Autodesk Inventor part; units mm, degrees
ref_plane "YZ Plane" through (0, 0, 0) normal (1, 0, 0) x (0, 1, 0)
ref_plane "XZ Plane" through (0, 0, 0) normal (0, 1, 0) x (-1, 0, 0)
ref_plane "XY Plane" through (0, 0, 0) normal (0, 0, 1) x (1, 0, 0)
sketch "Sketch1" plane through (0, 0, 0) normal (0, 0, 1) x (1, 0, 0)
  line L0 (0, 0) -> (43.269, 0)
  line L1 (43.269, 0) -> (43.269, 50)
  line L2 (43.269, 50) -> (50, 50)
  line L3 (50, 50) -> (50, 20)
  line L4 (50, 20) -> (43.269, 20)
  line L5 (43.269, 20) -> (43.269, 50)
  line L6 (3.269, 3.269) -> (23.269, 3.269)
  line L7 (23.269, 3.269) -> (23.269, 10)
  line L8 (23.269, 10) -> (3.269, 10)
  line L9 (3.269, 10) -> (3.269, 3.269)
  line L10 (0, 10) -> (3.269, 10)
  line L11 (23.269, 10) -> (43.269, 10)
  line L12 (43.269, 50) -> (40, 50)
  line L13 (0, 10) -> (0, 0)
  line L14 (0, 10) -> (0, 13.269)
  line L15 (0, 13.269) -> (40, 50)
  point P0 (13.269, 3.269)
  point P1 (13.269, 0)
  dimension "d2" = 30
  dimension "d3" = 20
  dimension "d5" = 6.731
  dimension "d6" = 10
  dimension "d9" = 3.269
  dimension "d11" = 20
  dimension "d12" = 20
  dimension "d14" = 3.269
  dimension "d15" = 3.269
extrude "Extrusion1" add sketch "Sketch1" along normal blind 6.731 contours L13 L10 L9 L6 L7 L11 L1 L0 | L14 L15 L12 L1 L11 L8 L10 | L1 L2 L3 L4
fillet "Fillet1" radius 2 3 edges at (40, 50, 3.3655) (0, 13.269, 3.3655) (0, 0, 3.3655)
equation "\"d5\" = THICKB"
equation "\"d7\" = THICKB"
equation "\"THICKA\" = 3.175"
equation "\"THICKB\" = 6.731"
equation "\"THICKC\" = 12.7"
equation "\"THICKPLY\" = 5"
equation "\"MAGDIA\" = 9.5"
equation "\"BALLDIA\" = 12"
properties part number "Mount_Mega_End"
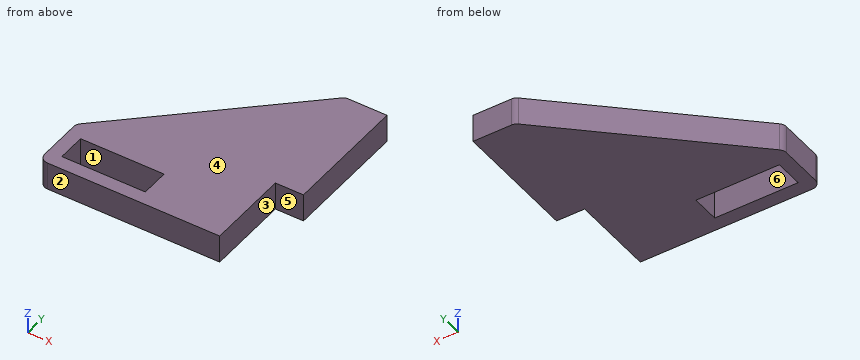
Can you work these out from the model? Positions are in its coordinate system, mm. Face numbers are marked on the shaded views. A direction names the side the tool comes from. Give positions to 0.01 mm unless a question says otherwise; leave off trailing zeros. Loops run counter-clockwise (first coordinate to the right, second up) from the corner with the lowest first, then second, coordinate; pieces in that order, holes last. Notation, with made-up numbers: (60, 39) - (116, 39) arc R4 cw to (116, 45) - close; hole circle Ø2 at (-35.5, 44). An arc over 180 degrees is marked (long way). Answer as a JSON object with one key per item and string values.
Q1. Will these pins go through, and if not, where does the flat tip stop? P1, Ø3.5, axis at y = 8, z = 2.5, coming from the +X side; P2, Ø3.5, axis at x = 17.5, z = 2.5, coming from the +Y side; P3, Ø12, axis at x = 6, y = 31.5, coming from the +Z side; P4, Ø4, axis at y = 20, z = 3, coming from the -X side.
Geometry says:
{"P1": "x = 43.27", "P2": "y = 30.95", "P3": "through", "P4": "x = 5.15"}
Q2. Imagine slicing it at A-A on z = 4.5. Write out the boundary of the cut face in (x, y).
Geometry says:
{"outline": "(0, 2) arc R2 ccw to (2, 0) - (43.27, 0) - (43.27, 20) - (50, 20) - (50, 50) - (40.78, 50) arc R2 ccw to (39.43, 49.47) - (0.65, 13.86) arc R2 ccw to (0, 12.39) - close; hole (3.27, 3.27) - (23.27, 3.27) - (23.27, 10) - (3.27, 10) - close"}
Q3. Imagine slicing it at D-D on x = 24.5. Write out the boundary of the cut face in (y, z).
Geometry says:
{"outline": "(0, 0) - (35.77, 0) - (35.77, 6.73) - (0, 6.73) - close"}
Q4. If I drill on L1, parallel to Y at x = 3.5, z = 1; L2, parallel to Y at x = 19.5, z = 1.25; L3, parallel to Y at x = 44, z = 5, over which ranges is the centre line in solid material (lowest first)?
Geometry says:
{"L1": "0 to 3.27, 10 to 16.48", "L2": "0 to 3.27, 10 to 31.18", "L3": "20 to 50"}
Q5. If we mould it in two halves opening along X, with no side actions, what happens to the marked faces 1, 2 and 3? For each: pulls with the +X half, pulls with the -X half, needs draft (parallel to the pull), parting line crosses it, or undercut.
Geometry says:
{"face 1": "undercut", "face 2": "needs draft", "face 3": "pulls with the +X half"}
Q6. Imagine slicing it at C-C on x = 4. Write out the boundary of the cut face in (y, z), plus the area to 3 significant figures.
Geometry says:
{"outline": "(0, 0) - (3.27, 0) - (3.27, 6.73) - (0, 6.73) - close; (10, 0) - (16.94, 0) - (16.94, 6.73) - (10, 6.73) - close", "area": "68.7 mm²"}
Q7. Imagine slicing it at B-B on y = 7. Write out the boundary of the cut face in (x, z), plus the area to 3 significant figures.
Geometry says:
{"outline": "(0, 0) - (3.27, 0) - (3.27, 6.73) - (0, 6.73) - close; (23.27, 0) - (43.27, 0) - (43.27, 6.73) - (23.27, 6.73) - close", "area": "157 mm²"}
Q8. Which directions (+Z, -Z, +X, -X, +Y, -Y) give clear straight access to the entire face, cutting with the end or side of a thin tool? Please do the marked faces 4, 5 and 6.
Geometry says:
{"face 4": "+Z, +X, -X, +Y, -Y", "face 5": "+Z, -Z, +X, -Y", "face 6": "+Z, -Z"}
